Autodesk Inventor part; units mm, degrees
ref_plane "YZ Plane" through (0, 0, 0) normal (1, 0, 0) x (0, 1, 0)
ref_plane "XZ Plane" through (0, 0, 0) normal (0, 1, 0) x (-1, 0, 0)
ref_plane "XY Plane" through (0, 0, 0) normal (0, 0, 1) x (1, 0, 0)
sketch "Sketch1" plane through (0, 0, 0) normal (0, 0, 1) x (1, 0, 0)
  line L0 (-25, 20) -> (25, 20)
  line L1 (25, 20) -> (25, 0)
  line L2 (-25, 0) -> (-25, 20)
  line L3 (-25, 0) -> (-5, 0)
  line L4 (-5, 0) -> (-5, 5)
  line L5 (-5, 5) -> (5, 5)
  line L6 (5, 5) -> (4.4322, 5)
  line L7 (5, 5) -> (5, 0)
  line L8 (5, 0) -> (25, 0)
  point P0 (0, 0)
  dimension "d0" = 50
  dimension "d1" = 20
  dimension "d3" = 25
  dimension "d4" = 20
  dimension "d5" = 5
  dimension "d6" = 10
  dimension "d7" = 5
  dimension "d8" = 20
extrude "Extrusion1" add sketch "Sketch1" along normal mid plane 20
properties part number "block"
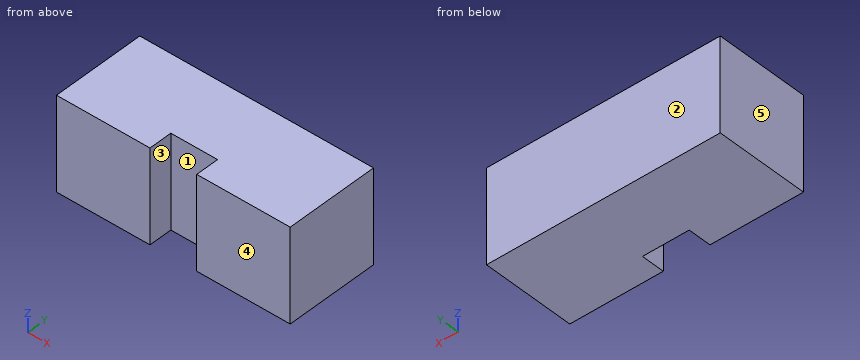
Part model, mm, in its own coordinate system. Face numbers are marked on the shaded views. A direction names the side the tool comes from. Give positions to 0.01 mm unless a question says otherwise; leave off trailing zeros. Write each loop counter-clockwise with the first axis right and the second up, starting at its lowest first coordinate (ties: lowest second). Pieces come first, ordered by that corner, then holes. Notation, with made-up numbers: (64.5, 26.25) -> (90.5, 26.25) arc R18 ccw to (90.5, 41.25) -> close; hole circle Ø11 at (16.5, 51.5). An arc over 180 degrees is marked (long way). Put each result on its own line as item: value. Start each with the question number.
Item 1: Pin check, flat tip, straight feed: pin 1 Ø5 at (x, z) = (0.5, 4) entering from -Y. Stop position of the tip, or through.
Item 2: Cut at C-C (x = -4). List the corners of the cut face in (y, z).
Item 3: Cut at A-A (y = 2.5). List the corners of the cut face in (x, z).
Item 4: Pull direction X, two halves, no side cores. Call the marked faces 3, 4 and 5: pulls with the +X half, pulls with the -X half, needs draft (parallel to the pull), parting line crosses it, or undercut.
Item 5: Which spindle directions (+Z, -Z, +X, -X, +Y, -Y) get a long thin tool onto all of the face, cutting with end or side? Do the marked faces 1 and 2. Say none if no direction does.
Item 6: Cut at B-B (z = -3.75). List the corners of the cut face in (x, y), then the cut area to 3 significant figures.
Item 7: Wall check: L1, parallel to X at y = 2.75, z = 0.75; L2, parallel to Y at x = -4, z = -2.75. Give the ranges that are in metal, low to high. Write a range as [from, to].
Answer list:
1. pin 1: stops at y = 5
2. outline: (5, -10) -> (20, -10) -> (20, 10) -> (5, 10) -> close
3. outline: (-25, -10) -> (-5, -10) -> (-5, 10) -> (-25, 10) -> close; (5, -10) -> (25, -10) -> (25, 10) -> (5, 10) -> close
4. face 3: undercut
4. face 4: needs draft
4. face 5: pulls with the -X half
5. face 1: +Z, -Z, -Y
5. face 2: +Z, -Z, +X, -X, +Y
6. outline: (-25, 0) -> (-5, 0) -> (-5, 5) -> (5, 5) -> (5, 0) -> (25, 0) -> (25, 20) -> (-25, 20) -> close
6. area: 950 mm2
7. L1: x = [-25, -5], [5, 25]
7. L2: y = [5, 20]
